Part model, mm, in its own coordinate system. Face numbers are marked on the shaded views. A direction names the side the tool comes from. Round coordinates to 2 decimals unless told otherwise and drop trailing zeros. Order: outer loops, then holes, each group sorted by start corner. A loop starts at its lowest first (then second) coordinate and runs counter-clockwise, first axis right, second up. Notation, with made-up numbers: (4, 45.5) -> (56, 45.5) arc R18 cw to (56, 71.5) -> close; hole circle Ø5 at (39, 58.25). An arc over 180 degrees is marked (long way). Return JSON: item names as keys, results as strings. Group by question number.
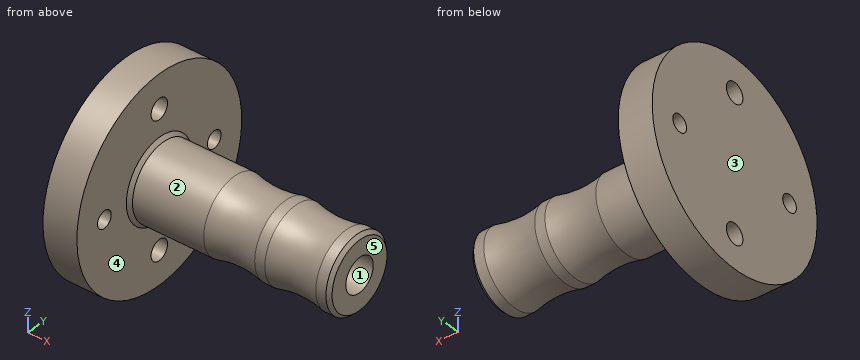
from build123d import *

# Parameters (mm, degrees)
F3_D     = 6
F5_D     = 5
F7_D     = 10
F7_DEPTH = 20
F7_TIP   = 3.0043030951


# Not quite as in the source:
# - a pattern or mirror of a feature is missing from the dataset's text; its kind, count and spacing are read off the source's solid


with BuildPart() as f1:
    # F0 (on Front) → F1 (revolve)
    with BuildSketch(Plane.XZ):
        with BuildLine():
            Line((-58, 11), (-59, 12))
            Line((-59, 12), (-59, 30))
            Line((-59, 30), (-69, 30))
            Line((-69, 30), (-69, 0))
            Line((-69, 0), (0, 0))
            Line((0, 0), (0, 10))
            Line((0, 10), (-1, 11))
            Line((-1, 11), (-4, 11))
            ThreePointArc((-4, 11), (-11.5, 10.0473750966), (-19, 11))
            Line((-19, 11), (-22, 11))
            ThreePointArc((-22, 11), (-29.5, 10.0473750966), (-37, 11))
            Line((-37, 11), (-58, 11))
        make_face()
    revolve(axis=Axis((-18.6788269784, 0, 0), (1, 0, 0)))

    # F3 (through all)
    with Locations(Plane(origin=(-69, 0, 0), x_dir=(0, -1, 0), z_dir=(-1, 0, 0))):
        with Locations((0, 20)):
            f3 = Hole(F3_D / 2)

    # F3_copies: F3 across plane
    add(f3.mirror(Plane(origin=(0, 0, 0), x_dir=(-1, 0, 0), z_dir=(0, 0, -1))), mode=Mode.SUBTRACT)

    # F5 (through all)
    with Locations(Plane(origin=(-69, 0, 0), x_dir=(0, -1, 0), z_dir=(-1, 0, 0))):
        with Locations((20, 0)):
            f5 = Hole(F5_D / 2)

    # F5_copies: F5 across plane
    add(f5.mirror(Plane.ZX), mode=Mode.SUBTRACT)

    # F7
    with Locations(Plane.YZ):
        with Locations((0, 0)):
            Hole(F7_D / 2, depth=F7_DEPTH)
            with Locations((0, 0, -(F7_DEPTH + F7_TIP / 2))):  # 118° drill point
                Cone(0, F7_D / 2, F7_TIP, mode=Mode.SUBTRACT)


solid = f1.part
(1) Pin check, flat tips, straight feed: P1, Ø10, axis at x = -54.5, z = -19, coming from the +Y side; P2, Ø8, axis at x = -43, y = -9.5, coming from the +Z side; P3, Ø5, axis at x = -59.5, y = 8, coming from the -Z side. Stop position of each tip, or through.
(2) Saw through at A-A, the plane x = -63. List the corners of the cut face in (y, z), and give its area (3 significant figures).
(3) Mould opens along Y. For the marked faces 1, 2 and 3 say: pulls with the +Y half, pulls with the -Y half, needs draft (parallel to the pull), parting line crosses it, or undercut.
(4) Saw through at C-C, the plane z = -20. List the corners of the cut face in (x, y).
(5) Tool access for the marked faces 4 and 5: list every direction of +Z, -Z, +X, -X, +Y, -Y with a clear straight run to the whole face (end or side of a thin tool).
(6) Saw through at D-D, the plane x = -41. List the corners of the cut face in (y, z), and give its area (3 significant figures).
(7) Saw through at B-B, the plane y = -20.5. List the corners of the cut face in (x, z), and give its area (3 significant figures).
(8) Probe L1, parallel to Z at x = -65, y = 0; L2, parallel to X at y = 4, z = -22.5; L3, parallel to Z at x = -12, y = 0. List the from-to ranges inside material, lowest first. Write a range as [from, to].
Results are:
{
 "1": {"P1": "stops at y = 24.84", "P2": "stops at z = 9.53", "P3": "stops at z = -29.49"},
 "2": {"outline": "circle Ø60 at (0, 0); hole circle Ø5 at (-20, 0); hole circle Ø6 at (0, -20); hole circle Ø6 at (0, 20); hole circle Ø5 at (20, 0)", "area": "2,730 mm^2"},
 "3": {"face 1": "undercut", "face 2": "parting line crosses it", "face 3": "needs draft"},
 "4": {"outline": "(-69, -22.36) -> (-59, -22.36) -> (-59, -3) -> (-69, -3) -> close; (-69, 3) -> (-59, 3) -> (-59, 22.36) -> (-69, 22.36) -> close"},
 "5": {"face 4": "+X", "face 5": "+Z, -Z, +X, +Y, -Y"},
 "6": {"outline": "circle Ø22 at (0, 0)", "area": "380 mm^2"},
 "7": {"outline": "(-69, -21.9) -> (-59, -21.9) -> (-59, -2.45) -> (-69, -2.45) -> close; (-69, 2.45) -> (-59, 2.45) -> (-59, 21.9) -> (-69, 21.9) -> close", "area": "389 mm^2"},
 "8": {"L1": "z = [-30, -23], [-17, 17], [23, 30]", "L2": "x = [-69, -59]", "L3": "z = [-10.05, -5], [5, 10.05]"}
}
